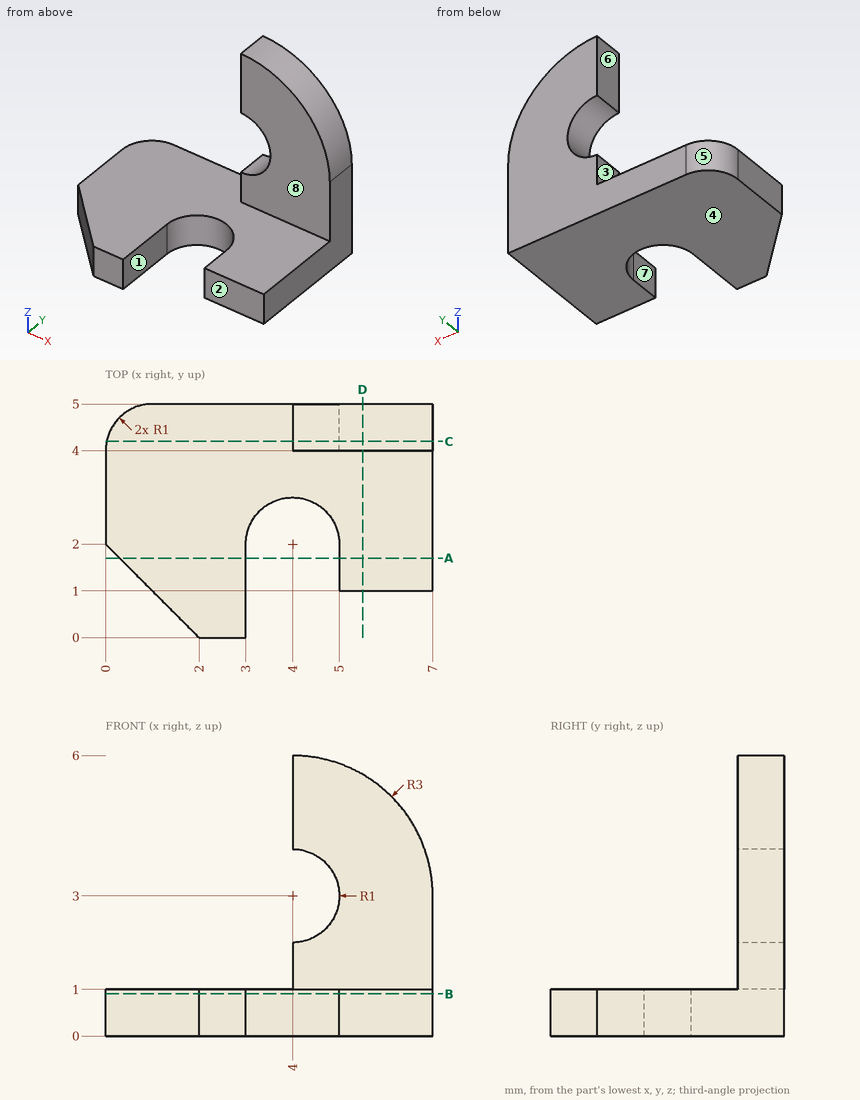
Drawing for the job (mm, zero at the part's lowest x, y, z). A direction names the side the tool comes from. Coordinates: 2 decimals unless noted, no trailing zeros. Write each loop counter-clockwise with the first axis right and the second up, starting at its lowest first coordinate (ties: lowest second). Pieces come first, ordered by that corner, then holes. Notation, with made-up numbers: (80, 6) -> (127, 6) arc R15 ccw to (127, 23) -> close; hole circle Ø11 at (-5, -31.5). An arc over 180 degrees is marked (long way). One line per item, written item: value. Start each with the question number.
1) Slice it at C-C on y = 4.2. Write the cut outline in (x, z), then the cut area to 3 significant figures.
2) Flat gauge pins, fed straight in: pin 1 Ø0.8 at (x, z) = (5.5, 0.5) entering from -Y; pin 2 Ø0.5 at (y, z) = (4.5, 1.5) entering from -X; pin 3 Ø2.5 at (x, y) = (5, 1.5) entering from +Z; pin 4 Ø1.5 at (y, z) = (1, 2) entering from +X. Where does each tip first touch, or does it go through?
3) Slice it at A-A on y = 1.7. Write the cut outline in (x, z), then the cut area to 3 significant figures.
4) Which spindle directions (+Z, -Z, +X, -X, +Y, -Y) get a long thin tool onto all of the face, cutting with end or side? Do the marked faces 1, 2, 3, 4 and 5. Say none if no direction does.
5) Slice it at B-B on z = 0.9. Write the cut outline in (x, y).
6) Probe probe 1 along Z at (x, y) = (0.5, 1.7); probe 2 along Y at (x, z) = (6, 1.45); probe 3 along Y at (x, z) = (6.25, 0.4). List the from-to ranges inside material, lowest first.
7) Pull direction X, two halves, no side cores. Call the marked faces 6, 7 and 8: +X half, -X half, draft (parallel to the pull), parting line (faces both ways), or undercut.
8) Slice it at D-D on x = 5.5. Write the cut outline in (y, z).
Answers follow:
1. outline: (0.02, 0) -> (7, 0) -> (7, 3) arc R3 ccw to (4, 6) -> (4, 4) arc R1 cw to (4, 2) -> (4, 1) -> (0.02, 1) -> close
1. area: 18.5 mm2
2. pin 1: y = 1
2. pin 2: x = 4
2. pin 3: z = 1
2. pin 4: through
3. outline: (0.3, 0) -> (3, 0) -> (3, 1) -> (0.3, 1) -> close; (5, 0) -> (7, 0) -> (7, 1) -> (5, 1) -> close
3. area: 4.70 mm2
4. face 1: +Z, -Z, -Y
4. face 2: +Z, -Z, +X, -Y
4. face 3: +Z, -X, +Y, -Y
4. face 4: -Z, +X, -X, +Y, -Y
4. face 5: +Z, -Z, -X, +Y
5. outline: (0, 2) -> (2, 0) -> (3, 0) -> (3, 2) arc R1 cw to (5, 2) -> (5, 1) -> (7, 1) -> (7, 5) -> (1, 5) arc R1 ccw to (0, 4) -> close
6. probe 1: 0 to 1
6. probe 2: 4 to 5
6. probe 3: 1 to 5
7. face 6: -X half
7. face 7: undercut
7. face 8: draft
8. outline: (1, 0) -> (5, 0) -> (5, 5.6) -> (4, 5.6) -> (4, 1) -> (1, 1) -> close
